```python
from build123d import *

# Parameters (mm, degrees)
F1_DEPTH = 38.1
F2_R     = 3.175
F3_DEPTH = 25.4
F4_R     = 6.35
F5_DEPTH = 25.4


with BuildPart() as f1:
    # F0 (on Front) → F1 (new body)
    with BuildSketch(Plane.XZ):
        Polygon((0, 69.85), (0, 0), (6.35, 0), (6.35, 76.2), (-44.45, 76.2), (-44.45, 69.85), align=None)
    extrude(amount=F1_DEPTH)

    # F2 (on face) → F3 (cut)
    with BuildSketch(Plane.YZ.offset(6.35)):
        with Locations((-19.05, 44.45)):
            Circle(F2_R)
        with Locations((-19.05, 19.05)):
            Circle(F2_R)
    extrude(amount=-F3_DEPTH, mode=Mode.SUBTRACT)

    # F4 (on face) → F5 (cut)
    with BuildSketch(Plane(origin=(0, 0, 69.85), x_dir=(1, 0, 0), z_dir=(0, 0, -1))):
        with Locations((-22.86, 19.05)):
            Circle(F4_R)
    extrude(amount=-F5_DEPTH, mode=Mode.SUBTRACT)


solid = f1.part
```
CAD build for the part. Positions are in the model's coordinates, mm. A direction names the side the tool comes from. Coordinates: 2 decimals unless noted, no trailing zeros. Order: outer loops, then holes, each group sorted by start corner. A loop starts at its lowest first (then second) coordinate and runs counter-clockwise, first axis right, second up.
(1) Saw through at C-C, the plane z = 45.5. Write the cut outline in (x, y).
Solution:
outline: (0, -38.1) - (6.35, -38.1) - (6.35, -22.05) - (0, -22.05) - close; (0, -16.05) - (6.35, -16.05) - (6.35, 0) - (0, 0) - close
(2) Which spindle directions (+Z, -Z, +X, -X, +Y, -Y) get a long thin tool onto all of the face, cutting with end or side? Do faces 1 (the face through (0, -19, 35)), 2 (the face through (3, -19, 0)). Say none if no direction does.
Solution:
face 1: -Z, -X, +Y, -Y
face 2: -Z, +X, -X, +Y, -Y
(3) Pin check, flat tips, straight feed: pin 1 Ø14.5 at (x, y) = (-22.86, -19.05) entering from +Z; pin 2 Ø19 at (y, z) = (-12, 51.5) entering from -X; pin 3 Ø6 at (x, y) = (-12, -6) entering from -Z. Stop position of each tip, or through.
Solution:
pin 1: stops at z = 76.2
pin 2: stops at x = 0
pin 3: stops at z = 69.85
(4) Saw through at D-D, the plane y = -23.5. Write the cut outline in (x, z), and give its area (3 significant figures).
Solution:
outline: (-44.45, 69.85) - (-27.39, 69.85) - (-27.39, 76.2) - (-44.45, 76.2) - close; (-18.33, 69.85) - (0, 69.85) - (0, 0) - (6.35, 0) - (6.35, 76.2) - (-18.33, 76.2) - close
area: 709 mm2
(5) Drill centre lines: L1, parallel to Z at x = 4, y = -19.05 (3 decimals); L2, parallel to Z at x = -1.5, y = -9; L3, parallel to X at y = -19, z = 30.5. Where is each one in solid material? Low to high.
Solution:
L1: z = 0 to 15.875, 22.225 to 41.275, 47.625 to 76.2
L2: z = 69.85 to 76.2
L3: x = 0 to 6.35
(6) Saw through at B-B, the plane y = -19.05. Write the cut outline in (x, z) (3 decimals).
Solution:
outline: (-44.45, 69.85) - (-29.21, 69.85) - (-29.21, 76.2) - (-44.45, 76.2) - close; (-16.51, 69.85) - (0, 69.85) - (0, 47.625) - (6.35, 47.625) - (6.35, 76.2) - (-16.51, 76.2) - close; (0, 0) - (6.35, 0) - (6.35, 15.875) - (0, 15.875) - close; (0, 22.225) - (6.35, 22.225) - (6.35, 41.275) - (0, 41.275) - close
(7) Mould opens along Z. For faces 3 (the face through (6.35, -19, 38)), 4 (the face through (3.219, -17.585, 16.233)), 5 (the face through (-13, -19, 76.2)) say: released by +Z, released by -Z, zero draft, split by the parting line, or undercut.
Solution:
face 3: zero draft
face 4: undercut
face 5: released by +Z
(8) Saw through at A-A, the plane x = -22.86. Write the cut outline in (y, z), and give its area (3 significant figures).
Solution:
outline: (-38.1, 69.85) - (-25.4, 69.85) - (-25.4, 76.2) - (-38.1, 76.2) - close; (-12.7, 69.85) - (0, 69.85) - (0, 76.2) - (-12.7, 76.2) - close
area: 161 mm2
